Here's the drawing with two shaded views (mm, measured from the low corner). I have some questions. A direction names the side the tool comes from. Give positions to 0.01 mm unless a question says otherwise; leave off trailing zeros. Write each loop counter-clockwise with the first axis right and the second up, starting at its lowest first coordinate (ties: lowest second). Pieces come first, ordered by that corner, then holes. Notation, with made-up numbers: (-33.5, 26.25) - (-6.5, 26.25) arc R7 ccw to (-6.5, 30.25) - close; hole circle Ø9 at (67, 17.5). An arc over 180 degrees is marked (long way). Write item = value, one per line.
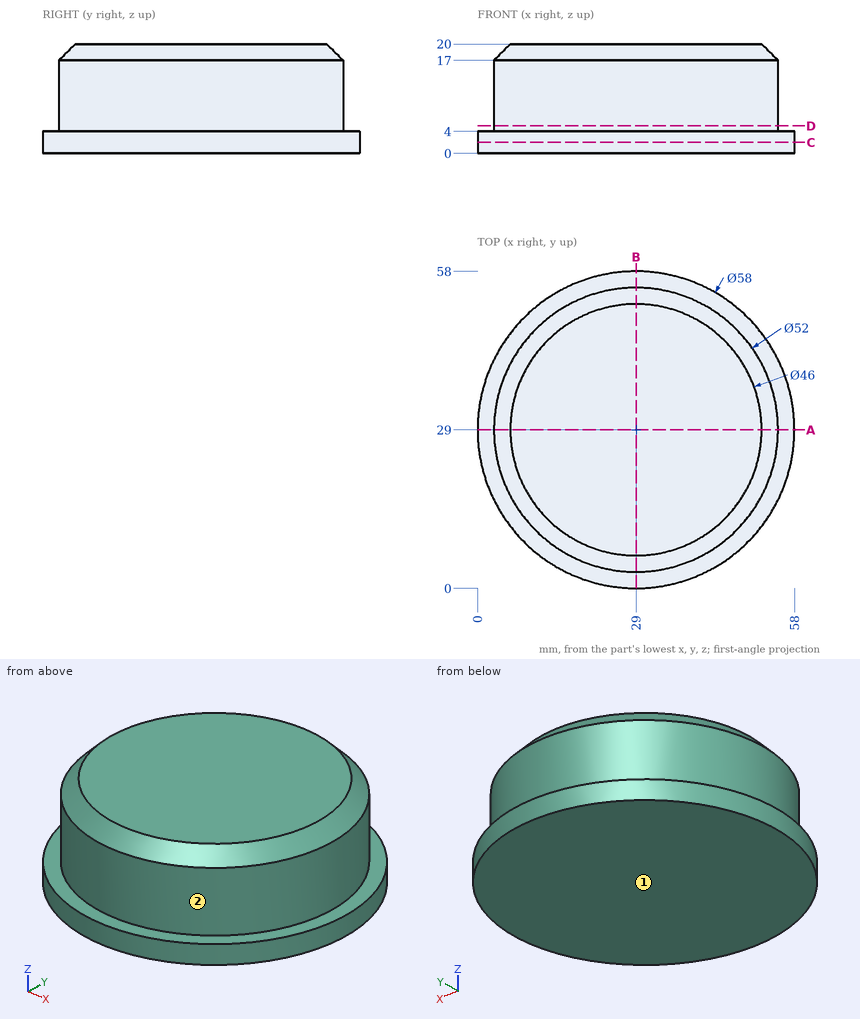
1. Which directions (+Z, -Z, +X, -X, +Y, -Y) give clear straight access to the entire face, cutting with the end or side of a thin tool? Please do the marked faces 1 and 2.
Filled sheet:
face_1 = -Z, +X, -X, +Y, -Y
face_2 = +Z
2. If we section it at A-A, the plane y = 29: Please give me the cut outline in (x, z).
Filled sheet:
outline = (0, 0) - (58, 0) - (58, 4) - (55, 4) - (55, 17) - (52, 20) - (6, 20) - (3, 17) - (3, 4) - (0, 4) - close
3. For pin 1 (1 mm diameter, centred on x = 36, z = 2.5, fed in from +Y); pin 2 (6 mm diameter, centred on y = 18.5, z = 14.5, fed in from -X); pin 3 (10 mm diameter, centred on x = 38.5, z = 6.5, fed in from +Y), each with a flat end and sliding along its axis, tell me the tip position at first contact or that it passes through.
Filled sheet:
pin_1 = 57.26
pin_2 = 4.11
pin_3 = 57.54
4. If we section it at C-C, the plane z = 2: Please give me the cut outline in (x, y), and give its area (3 significant figures).
Filled sheet:
outline = circle Ø58 at (29, 29)
area = 2,640 mm2
5. I need wall thicknesses on line 1 (Y direction, x = 29.5, z = 5); line 2 (Z direction, x = 5.5, y = 25.5); line 3 (Y direction, x = 14, z = 8). Which ranges of each line are inside material? Lowest first, please.
Filled sheet:
line_1 = 3 to 55
line_2 = 0 to 19.24
line_3 = 7.76 to 50.24
6. If we section it at D-D, the plane z = 5: Please give me the cut outline in (x, y), and give its area (3 significant figures).
Filled sheet:
outline = circle Ø52 at (29, 29)
area = 2,120 mm2
